```python
from build123d import *

# Parameters (mm, degrees)
BOSS_EXTRUDE1_DEPTH = 29.4
SKETCH2_R           = 18.5
CUT_EXTRUDE1_DEPTH  = 6.85
SKETCH3_R           = 2.5
BOSS_EXTRUDE2_DEPTH = 12.35
SKETCH4_R           = 2.85
BOSS_EXTRUDE3_DEPTH = 4
CUT_EXTRUDE3_DEPTH  = 7
SKETCH6_R           = 1.5
CUT_EXTRUDE4_DEPTH  = 40.8
SKETCH7_R           = 1
CUT_EXTRUDE5_DEPTH  = 35.9


with BuildPart() as part:
    # Sketch1 → Boss-Extrude1 (new body)
    with BuildSketch(Plane(origin=(0, 0, 0), x_dir=(1, 0, 0), z_dir=(0, 1, 0))):
        with BuildLine():
            Line((-13.950766, 19.9), (21.950766, 19.9))
            ThreePointArc((21.950766, 19.9), (30.8, 0), (21.950766, -19.9))
            Line((21.950766, -19.9), (-13.950766, -19.9))
            ThreePointArc((-13.950766, -19.9), (-18.785456749, -14.108967388), (-21.81472448, -7.2))
            Line((-21.81472448, -7.2), (-26.15, -7.2))
            ThreePointArc((-26.15, -7.2), (-27.917766953, -6.467766953), (-28.65, -4.7))
            Line((-28.65, -4.7), (-28.65, 14))
            ThreePointArc((-28.65, 14), (-27.917766953, 15.767766953), (-26.15, 16.5))
            Line((-26.15, 16.5), (-17.118475324, 16.5))
            ThreePointArc((-17.118475324, 16.5), (-15.608452372, 18.268787469), (-13.950766, 19.9))
        make_face()
    extrude(amount=BOSS_EXTRUDE1_DEPTH)

    # Sketch2 → Cut-Extrude1 (cut)
    with BuildSketch(Plane(origin=(0, 29.4, 0), x_dir=(1, 0, 0), z_dir=(0, 1, 0))):
        Circle(SKETCH2_R)
    extrude(amount=-CUT_EXTRUDE1_DEPTH, mode=Mode.SUBTRACT)

    # Sketch3 → Boss-Extrude2 (add)
    with BuildSketch(Plane(origin=(0, 22.55, 0), x_dir=(1, 0, 0), z_dir=(0, 1, 0))):
        Circle(SKETCH3_R)
    extrude(amount=BOSS_EXTRUDE2_DEPTH)

    # Sketch4 → Boss-Extrude3 (add)
    with BuildSketch(Plane.XZ):
        Circle(SKETCH4_R)
    extrude(amount=BOSS_EXTRUDE3_DEPTH)

    # Sketch5 → Cut-Extrude3 (cut)
    with BuildSketch(Plane(origin=(0, 29.4, 0), x_dir=(1, 0, 0), z_dir=(0, 1, 0))):
        with BuildLine():
            Line((-29.993194127, 17.400116254), (-16.38322728, 17.400116254))
            ThreePointArc((-16.38322728, 17.400116254), (-22.242311501, 5.438849795), (-21.619709811, -7.86577836))
            Line((-21.619709811, -7.86577836), (-29.993194127, -7.86577836))
            Line((-29.993194127, -7.86577836), (-29.993194127, 17.400116254))
        make_face()
    extrude(amount=-CUT_EXTRUDE3_DEPTH, mode=Mode.SUBTRACT)

    # Sketch6 → Cut-Extrude4 (cut, through all)
    with BuildSketch(Plane.XY.offset(19.9)):
        with Locations((-3.85, 14.7)):
            Circle(SKETCH6_R)
        with Locations((10.85, 14.7)):
            Circle(SKETCH6_R)
    extrude(amount=-CUT_EXTRUDE4_DEPTH, mode=Mode.SUBTRACT)

    # Sketch7 → Cut-Extrude5 (cut, through all)
    with BuildSketch(Plane.XZ):
        with Locations((-13.833383534, 15.6)):
            Circle(SKETCH7_R)
        with Locations((22.22970985, 15.5)):
            Circle(SKETCH7_R)
        with Locations((22.22970985, -15.5)):
            Circle(SKETCH7_R)
        with Locations((-9.553140845, -17.4)):
            Circle(SKETCH7_R)
    extrude(amount=-CUT_EXTRUDE5_DEPTH, mode=Mode.SUBTRACT)


solid = part.part
```
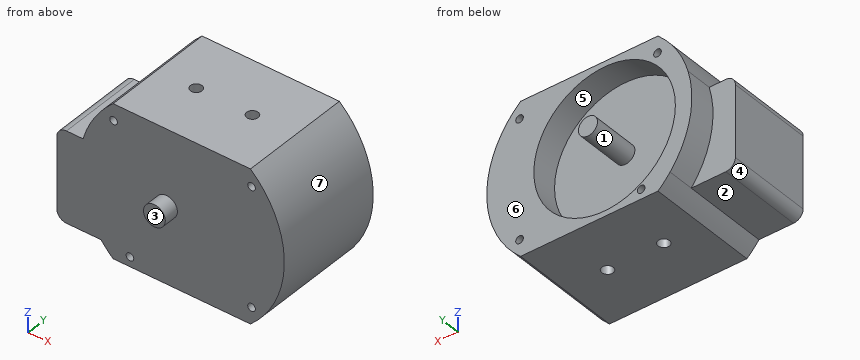
Geometry check sheet. Reference: the model listing, model coordinates, mm. Face numbers are marked on the shaded views. A direction names the side the tool comes from. Give positions to 0.01 mm unless a question says otherwise; leave off trailing zeros. Order: outer loops, then holes, each group sorted by start corner. A loop starts at its lowest first (then second) coordinate and runs counter-clockwise, first axis right, second up. Notation, with made-up numbers: (69, 73.5) - (88, 73.5) arc R21 ccw to (88, 82.5) - close; hole circle Ø1 at (53.25, 64.5). An arc over 180 degrees is marked (long way). Write item = value, one per line. Start each with the question number.
1) Section check B-B (z = 0). Enter the section's corners in (x, y).
2) Scan lines: L1, parallel to Y at x = 11, z = -12.5; L2, parallel to Z at x = 22, y = 14.5; L3, parallel to Z at x = -10, y = 23.5. Record each from-to range of solid material in increasing order.
3) Section check C-C (x = 10.85). Enter the section's corners in (y, z).
4) Draft check along Z on the marked faces 4, 5, 6 and 7. Enter one of: released by +Z, released by -Z, zero draft, split by the parting line, or undercut.
5) Gauge pin test, flat ends, axial feed: pin 1 Ø2.5 at (x, y) = (-20.5, 13) entering from -Z; pin 2 Ø12.5 at (x, z) = (-23.5, -5) entering from +Y; pin 3 Ø4 at (x, z) = (-10, 1.5) entering from -Y. Record the tip position at first contact, or that the pin passes through.
6) Access from +Z, -Z, +X, -X, +Y, -Y to the whole of each face (thin tool, end or side, straight path). Record for the marked faces 1, 2 and 3.
7) Section check A-A (y = 18). Enter the section's corners in (x, z).
8) Section check D-D (y = 14). Enter the section's corners in (x, z), then the cut area to 3 significant figures.
Geometry check:
q1.outline = (-28.65, 0) - (-2.85, 0) - (-2.85, -4) - (2.85, -4) - (2.85, 0) - (30.8, 0) - (30.8, 29.4) - (18.5, 29.4) - (18.5, 22.55) - (2.5, 22.55) - (2.5, 34.9) - (-2.5, 34.9) - (-2.5, 22.55) - (-18.5, 22.55) - (-18.5, 29.4) - (-22.8, 29.4) - (-22.8, 22.4) - (-28.65, 22.4) - close; hole circle Ø3 at (-3.85, 14.7); hole circle Ø3 at (10.85, 14.7)
q2.L1 = 0 to 13.21, 16.19 to 22.55
q2.L2 = -19.86 to -16.47, -14.53 to 14.53, 16.47 to 19.86
q2.L3 = -19.9 to -18.29, -16.51 to -15.56, 15.56 to 19.9
q3.outline = (0, -19.9) - (13.2, -19.9) - (13.2, 19.9) - (0, 19.9) - close; (16.2, -19.9) - (29.4, -19.9) - (29.4, -14.98) - (22.55, -14.98) - (22.55, 14.98) - (29.4, 14.98) - (29.4, 19.9) - (16.2, 19.9) - close
q4.face_4 = released by -Z
q4.face_5 = undercut
q4.face_6 = zero draft
q4.face_7 = split by the parting line
q5.pin_1 = -16.5
q5.pin_2 = 29.4
q5.pin_3 = 0
q6.face_1 = +Y
q6.face_2 = -Z, -X, +Y, -Y
q6.face_3 = +Z, -Z, +X, -X, -Y
q7.outline = (-28.65, -14) arc R2.5 ccw to (-26.15, -16.5) - (-17.12, -16.5) arc R26.8 ccw to (-13.95, -19.9) - (21.95, -19.9) arc R26.8 ccw to (21.95, 19.9) - (-13.95, 19.9) arc R26.8 ccw to (-21.81, 7.2) - (-26.15, 7.2) arc R2.5 ccw to (-28.65, 4.7) - close; hole circle Ø2 at (-13.83, 15.6); hole circle Ø2 at (-9.55, -17.4); hole circle Ø2 at (22.23, -15.5); hole circle Ø2 at (22.23, 15.5)
q8.outline = (-28.65, -14) arc R2.5 ccw to (-26.15, -16.5) - (-17.12, -16.5) arc R26.8 ccw to (-13.95, -19.9) - (-5.18, -19.9) - (-5.18, 19.9) - (-13.95, 19.9) arc R26.8 ccw to (-21.81, 7.2) - (-26.15, 7.2) arc R2.5 ccw to (-28.65, 4.7) - close; (-2.52, -19.9) - (9.52, -19.9) - (9.52, 19.9) - (-2.52, 19.9) - close; (12.18, -19.9) - (21.95, -19.9) arc R26.8 ccw to (21.95, 19.9) - (12.18, 19.9) - close; hole circle Ø2 at (-13.83, 15.6); hole circle Ø2 at (-9.55, -17.4); hole circle Ø2 at (22.23, -15.5); hole circle Ø2 at (22.23, 15.5)
q8.area = 1,860 mm2
